Work out the finished part from the listing and answer in its coordinate system (mm). A direction names the side the tool comes from. Round coordinates to 2 decimals unless told otherwise and drop trailing zeros. Order: outer loops, then holes, each group sorted by start corner. A loop starts at its lowest first (then second) coordinate and runs counter-clockwise, first axis right, second up. Notation, with made-up numbers: (84.5, 4) - (91.5, 4) arc R15 ccw to (91.5, 23) - close; hole circle Ø4 at (82.5, 22.25). An arc over 180 degrees is marked (long way). Answer in a Markdown table with one row per item.
from build123d import *

# Parameters (mm, degrees)
F1_DEPTH = 140
F2_DEPTH = 137
F3_DEPTH = 5
F4_W     = 4.0531810373
F4_H     = 6.6223293543
F5_DEPTH = 5
F7_DEPTH = 12
F9_DEPTH = 31
F10_R    = 5
F11_R    = 2
F12_R    = 2
F13_R    = 5


with BuildPart() as f1:
    # F0 (on Top) → F1 (new body)
    with BuildSketch(Plane.XY):
        with BuildLine():
            Line((-37, 47.5), (-37, 37))
            Line((-37, 37), (-47.5, 37))
            ThreePointArc((-47.5, 37), (-67, 17.5), (-47.5, -2))
            Line((-47.5, -2), (2, -2))
            Line((2, -2), (2, 47.5))
            ThreePointArc((2, 47.5), (-17.5, 67), (-37, 47.5))
        make_face()
        with BuildLine():
            Line((0, 47.5), (0, 0))
            Line((0, 0), (-47.5, 0))
            ThreePointArc((-47.5, 0), (-65, 17.5), (-47.5, 35))
            Line((-47.5, 35), (-35, 35))
            Line((-35, 35), (-35, 47.5))
            ThreePointArc((-35, 47.5), (-17.5, 65), (0, 47.5))
        make_face(mode=Mode.SUBTRACT)
    extrude(amount=F1_DEPTH)

    # F0 (on Top) → F2 (join)
    with BuildSketch(Plane.XY):
        with BuildLine():
            Line((-47.5, 0), (0, 0))
            Line((0, 0), (0, 47.5))
            ThreePointArc((0, 47.5), (-17.5, 65), (-35, 47.5))
            Line((-35, 47.5), (-35, 35))
            Line((-35, 35), (-47.5, 35))
            ThreePointArc((-47.5, 35), (-65, 17.5), (-47.5, 0))
        make_face()
        with BuildLine():
            Line((-47.5, 32), (-32, 32))
            Line((-32, 32), (-32, 47.5))
            ThreePointArc((-32, 47.5), (-17.5, 62), (-3, 47.5))
            Line((-3, 47.5), (-3, 3))
            Line((-3, 3), (-47.5, 3))
            ThreePointArc((-47.5, 3), (-62, 17.5), (-47.5, 32))
        make_face(mode=Mode.SUBTRACT)
    extrude(amount=F2_DEPTH)

    # F0 (on Top) → F3 (join)
    with BuildSketch(Plane.XY):
        with BuildLine():
            Line((-32, 47.5), (-32, 32))
            Line((-32, 32), (-47.5, 32))
            ThreePointArc((-47.5, 32), (-62, 17.5), (-47.5, 3))
            Line((-47.5, 3), (-3, 3))
            Line((-3, 3), (-3, 47.5))
            ThreePointArc((-3, 47.5), (-17.5, 62), (-32, 47.5))
        make_face()
    extrude(amount=F3_DEPTH)

    # F4 (on face) → F5 (join)
    with BuildSketch(Plane.YZ.offset(2)):
        with Locations((19.9135849252, 105.5362299085)):
            Rectangle(F4_W, F4_H)
    extrude(amount=F5_DEPTH)

    # F6 (on face) → F7 (join)
    with BuildSketch(Plane.XZ.offset(-17.8869944066)):
        with BuildLine():
            Line((12.1471862551, 118.9945808407), (2, 108.8473945856))
            Line((2, 108.8473945856), (2, 102.2250652313))
            Line((2, 102.2250652313), (5.5355339059, 105.3118606797))
            Line((5.5355339059, 105.3118606797), (15.682720161, 115.4590469347))
            ThreePointArc((15.682720161, 115.4590469347), (36.8959235966, 115.4590469347), (36.8959235966, 94.2458434991))
            Line((36.8959235966, 94.2458434991), (2, 59.3499199026))
            Line((2, 59.3499199026), (2, 52.2788520907))
            Line((2, 52.2788520907), (40.4314575025, 90.7103095932))
            ThreePointArc((40.4314575025, 90.7103095932), (40.4314575025, 118.9945808407), (12.1471862551, 118.9945808407))
        make_face()
    extrude(amount=-F7_DEPTH)

    # F8 (on face) → F9 (cut)
    with BuildSketch(Plane.XZ.offset(-17.8869944066)):
        Polygon((7, 102.2250652313), (7, 106.7763267737), (2, 102.2250652313), align=None)
    extrude(amount=-F9_DEPTH, mode=Mode.SUBTRACT)

    # F10
    f10_edges = [f1.edges().sort_by_distance(p)[0] for p in [
        (-62, 17.5, 5),
        (-32, 39.75, 5),
        (-3, 3, 71),
    ]]
    fillet(f10_edges, radius=F10_R)

    # F11
    f11_edges = [f1.edges().sort_by_distance(p)[0] for p in [
        (40.431458, 17.886994, 118.994581),
        (7.073593, 17.886994, 113.920988),
        (21.215729, 17.886994, 71.494581),
        (36.895924, 17.886994, 115.459047),
        (11.34136, 17.886994, 111.117687),
        (4.5, 17.886994, 104.500696),
        (19.447962, 17.886994, 76.797882),
        (21.215729, 29.886994, 71.494581),
        (40.431458, 29.886994, 118.994581),
        (19.447962, 29.886994, 76.797882),
        (36.895924, 29.886994, 115.459047),
        (11.34136, 29.886994, 111.117687),
        (4.5, 29.886994, 104.500696),
        (7.073593, 29.886994, 113.920988),
    ]]
    fillet(f11_edges, radius=F11_R)

    # F12
    f12_edges = [f1.edges().sort_by_distance(p)[0] for p in [
        (2, -2, 70),
    ]]
    fillet(f12_edges, radius=F12_R)

    # F13
    f13_edges = [f1.edges().sort_by_distance(p)[0] for p in [
        (0, 0, 138.5),
    ]]
    fillet(f13_edges, radius=F13_R)


solid = f1.part
1) The mould has two halves that part along X. Classify faces 5 (the face through (11.281, 23.831, 111.057)), 6 (the face through (-35.2, 35.2, 140)), 7 (the face through (20.95, 23.83, 71.23)), 8 (the face through (-37, 42, 69)): released by +X, released by -X, zero draft, split by the parting line, or undercut.
Filled in:
| item | result |
|---|---|
| face 5 | undercut |
| face 6 | zero draft |
| face 7 | released by +X |
| face 8 | released by -X |
2) Which of the six approach directions +Z, -Z, +X, -X, +Y, -Y give full straight-line access (tool end or side, diameter ignored) to faces 1 (the face through (32.4, 17.887, 86.6)), 2 (the face through (18.89, 18.488, 75.433)), 3 (the face through (-24, -2, 69)), 4 (the face through (-3, 28, 73))?
Filled in:
| item | result |
|---|---|
| face 1 | +Z, -Z, +X, -Y |
| face 2 | -Y |
| face 3 | +Z, -Z, +X, -X, -Y |
| face 4 | +Z |
3) Find section D-D, the plane x = -44. Give the vertices of the cut face in (y, z), then the cut area to 3 significant figures.
Filled in:
| item | result |
|---|---|
| outline | (-2, 0) - (37, 0) - (37, 140) - (35, 140) - (35, 137) - (32, 137) - (32, 10) arc R5 cw to (27, 5) - (8, 5) arc R5 cw to (3, 10) - (3, 137) - (0, 137) - (0, 140) - (-2, 140) - close |
| area | 1,540 mm^2 |
4) Find the intervals of material crossed by probe 1 along Y at (x, z) = (-44, 50); probe 2 along Y at (x, z) = (-17, 91); probe 3 along X at (y, z) = (18, 129), in increasing order. Write a range as from..to.
Filled in:
| item | result |
|---|---|
| probe 1 | y = -2..3, 32..37 |
| probe 2 | y = -2..3, 61.99..66.99 |
| probe 3 | x = -66.99..-61.99, -3..2 |
5) Find section A-A, the plane z = 21. Give the vertices of the cut face in (x, y).
Filled in:
| item | result |
|---|---|
| outline | (-47.5, -2) - (0, -2) arc R2 ccw to (2, 0) - (2, 47.5) arc R19.5 ccw to (-37, 47.5) - (-37, 37) - (-47.5, 37) arc R19.5 ccw to start; hole (-47.5, 3) - (-8, 3) arc R5 ccw to (-3, 8) - (-3, 47.5) arc R14.5 ccw to (-32, 47.5) - (-32, 32) - (-47.5, 32) arc R14.5 ccw to start |
6) Find section B-B, the plane x = -17.5. Give the vertices of the cut face in (y, z).
Filled in:
| item | result |
|---|---|
| outline | (-2, 0) - (67, 0) - (67, 140) - (65, 140) - (65, 137) - (62, 137) - (62, 10) arc R5 cw to (57, 5) - (8, 5) arc R5 cw to (3, 10) - (3, 137) - (0, 137) - (0, 140) - (-2, 140) - close |
7) Each of these flat-tipped pins is pushed along its axis until it touches: pin 1 (12 mm diameter, centred on x = 6, z = 107, fed in from +Y); pin 2 (2 mm diameter, centred on x = -43, y = 14, fed in from +Z); pin 3 (0.9 mm diameter, centred on y = 41, z = 138.5, fed in from +X). Where does it stop, or does it pass through?
Filled in:
| item | result |
|---|---|
| pin 1 | stops at y = 56.1 |
| pin 2 | stops at z = 5 |
| pin 3 | stops at x = 2 |
8) Find section C-C, the plane z = 64. Give the number of separate pieces and of enclosed holes in the cut face, then the cut area to 3 significant figures.
Filled in:
| item | result |
|---|---|
| separate pieces | 2 |
| enclosed holes | 1 |
| area | 1,220 mm^2 |
